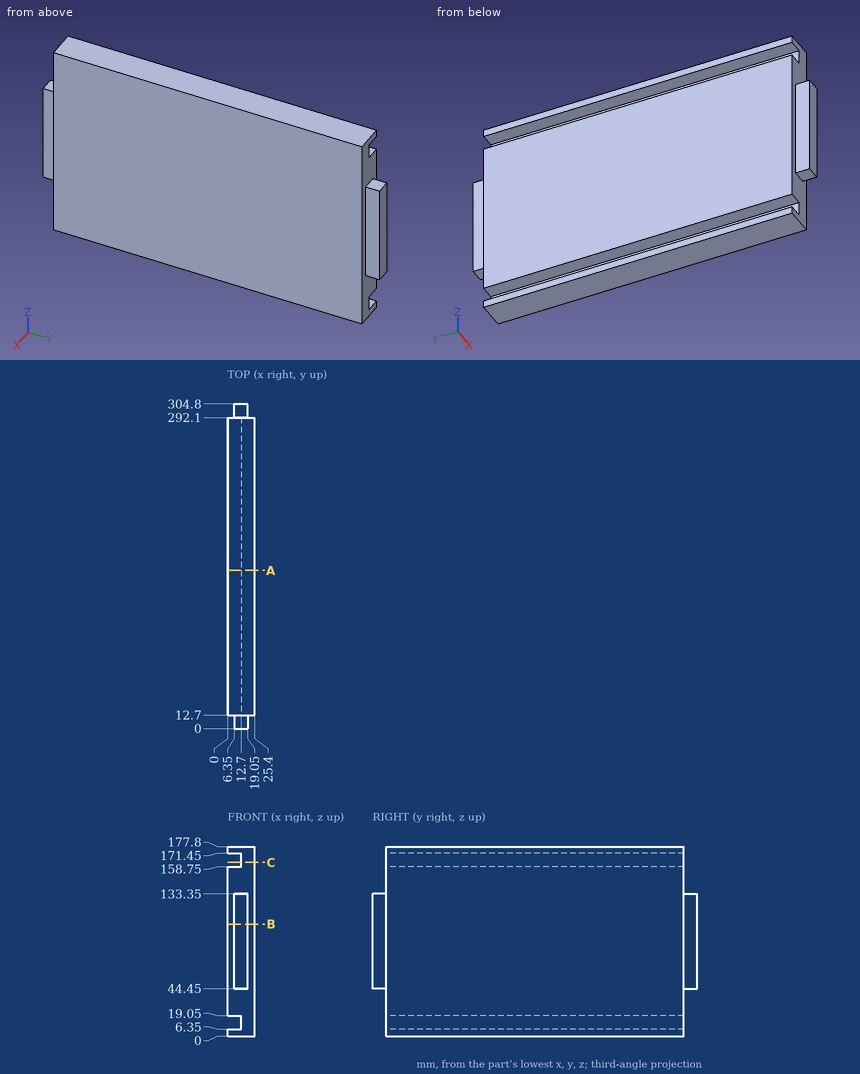
Input: dimensioned drawing with shaded views. Units: mm. Origin: part minimum x, y, z. Coordinates: 2 decimals unless noted, no trailing zeros. Loops run counter-clockwise (first coordinate to the right, second up) from the corner with the lowest first, then second, coordinate; pieces in that order, holes last. Notation, with made-up numbers: M 60.25,16 L 104.25,16 A27 ccw 104.25,35 Z; hole C 41.25,9 d2. An arc over 180 degrees is marked long. One line per item, written item: value.
(1) Section B-B (z = 105). Output: boundary loops of the cut face in (x, y), and give its area (3 significant figures).
Filled in:
outline: M 0,12.7 L 6.35,12.7 L 6.35,0 L 19.05,0 L 19.05,12.7 L 25.4,12.7 L 25.4,292.1 L 19.05,292.1 L 19.05,304.8 L 6.35,304.8 L 6.35,292.1 L 0,292.1 Z
area: 7,420 mm^2
(2) Section C-C (z = 163). Output: boundary loops of the cut face in (x, y).
Filled in:
outline: M 12.7,12.7 L 25.4,12.7 L 25.4,292.1 L 12.7,292.1 Z
(3) Section A-A (y = 148.5). Output: boundary loops of the cut face in (x, z).
Filled in:
outline: M 0,0 L 25.4,0 L 25.4,177.8 L 0,177.8 L 0,171.45 L 12.7,171.45 L 12.7,158.75 L 0,158.75 L 0,19.05 L 12.7,19.05 L 12.7,6.35 L 0,6.35 Z
(4) Pin query (flat end, axial travel): pin 1 (10 mm diameter, centred on y = 145.5, z = 12.5, fed in from -X); pin 2 (5 mm diameter, centred on x = 20, z = 144, fed in from -Y); pin 3 (4 mm diameter, centred on y = 6.5, z = 83, fed in from -X). Return the tip coordinate at first contact, or that it passes through.
Filled in:
pin 1: x = 12.7
pin 2: y = 12.7
pin 3: x = 6.35
(5) Line query: line 1 along Z through (x, y) = (7.25, 258); line 2 along Y through (x, z) = (5.25, 100.5); line 3 along X through (y, z) = (186.5, 9). Output: solid intervals per line, ascending. Write a range as from..to.
Filled in:
line 1: 0..6.35, 19.05..158.75, 171.45..177.8
line 2: 12.7..292.1
line 3: 12.7..25.4
